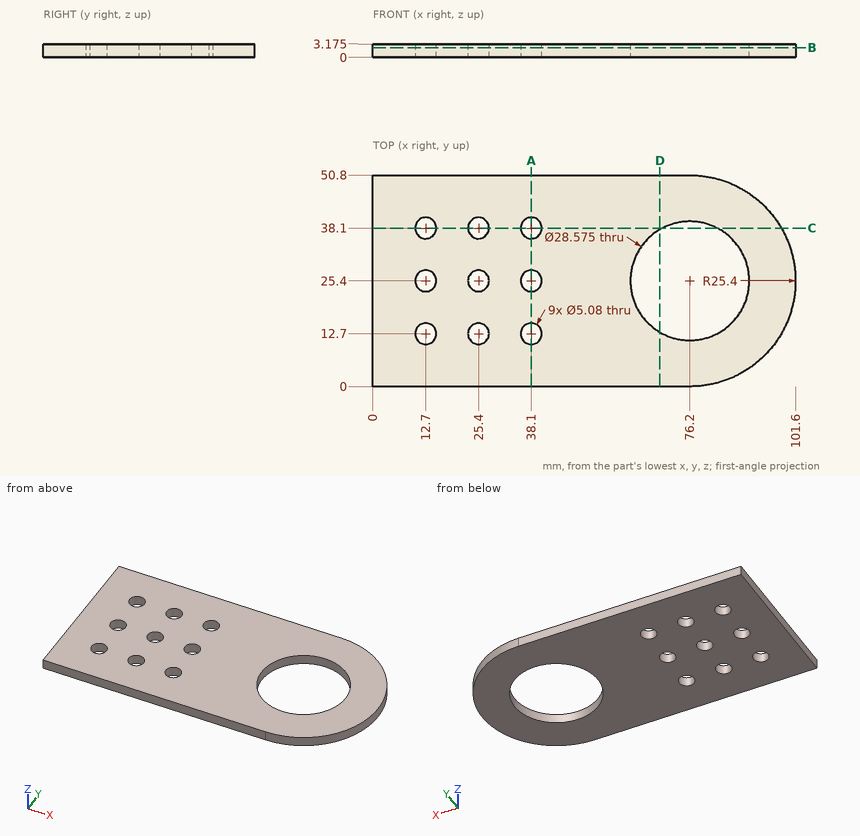
Job drawing, mm, ordinate dimensions from the low corner. One solid piece. Give positions to 0.01 mm unless a question says otherwise; leave off trailing zeros. Loops run counter-clockwise (first coordinate to the right, second up) from the corner with the lowest first, then second, coordinate; pieces in that order, holes last. Notation, with made-up numbers: M -28.5,67 L 28.5,67 A15 cw 28.5,84 Z; hole C -29,77 d2. An arc over 180 degrees is marked long. Answer in a Markdown table with one row per item. Add a question column.
Item 1: Probe probe 1 along Y at (x, z) = (38.1, 2.2); probe 2 along X at (y, z) = (27.5, 1.75); probe 3 along X at (y, z) = (36, 0.3). List the from-to ranges inside material, lowest first.
Item 2: Band-saw the part on D-D on x = 69. Give the cut face in (y, z) (3 decimals), then the cut area to 3 significant figures.
Item 3: Band-saw the part on B-B on z = 2.3. Give the number of separate pieces and of enclosed holes in the cut face, then the cut area to 3 significant figures.
Item 4: Band-saw the part on C-C on y = 38.1. Give the cut face in (x, z) (3 decimals).
Item 5: Band-saw the part on A-A on x = 38.1. Give the cut face in (y, z) (3 decimals), then the cut area to 3 significant figures.
Reply:
| question | item | result |
|---|---|---|
| 1 | probe 1 | y = 0 to 10.16, 15.24 to 22.86, 27.94 to 35.56, 40.64 to 50.8 |
| 1 | probe 2 | x = 0 to 11.27, 14.13 to 23.97, 26.83 to 36.67, 39.53 to 62.07, 90.33 to 101.51 |
| 1 | probe 3 | x = 0 to 11.27, 14.13 to 23.97, 26.83 to 36.67, 39.53 to 66.62, 85.78 to 99.28 |
| 2 | outline | M 0,0 L 13.059,0 L 13.059,3.175 L 0,3.175 Z; M 37.741,0 L 50.8,0 L 50.8,3.175 L 37.741,3.175 Z |
| 2 | area | 82.9 mm^2 |
| 3 | separate pieces | 1 |
| 3 | enclosed holes | 10 |
| 3 | area | 4,060 mm^2 |
| 4 | outline | M 0,0 L 10.16,0 L 10.16,3.175 L 0,3.175 Z; M 15.24,0 L 22.86,0 L 22.86,3.175 L 15.24,3.175 Z; M 27.94,0 L 35.56,0 L 35.56,3.175 L 27.94,3.175 Z; M 40.64,0 L 69.655,0 L 69.655,3.175 L 40.64,3.175 Z; M 82.745,0 L 98.197,0 L 98.197,3.175 L 82.745,3.175 Z |
| 5 | outline | M 0,0 L 10.16,0 L 10.16,3.175 L 0,3.175 Z; M 15.24,0 L 22.86,0 L 22.86,3.175 L 15.24,3.175 Z; M 27.94,0 L 35.56,0 L 35.56,3.175 L 27.94,3.175 Z; M 40.64,0 L 50.8,0 L 50.8,3.175 L 40.64,3.175 Z |
| 5 | area | 113 mm^2 |
